```python
from build123d import *

# Parameters (mm, degrees)
BOSS_EXTRUDE1_DEPTH = 2


with BuildPart() as part:
    # Sketch1 → Boss-Extrude1 (new body)
    with BuildSketch(Plane(origin=(0, 0, 0), x_dir=(0, 0, -1), z_dir=(1, 0, 0))):
        with BuildLine():
            Line((-18, 0), (-15, 0))
            Line((-15, 0), (-15, 2))
            Line((-15, 2), (-5, 2))
            Line((-5, 2), (-5, 0))
            Line((-5, 0), (5, 0))
            Line((5, 0), (5, 2))
            Line((5, 2), (15, 2))
            Line((15, 2), (15, 0))
            Line((15, 0), (18, 0))
            Line((18, 0), (18, -2))
            Line((18, -2), (20, -2))
            Line((20, -2), (20, -12))
            Line((20, -12), (18, -12))
            Line((18, -12), (18, -15))
            ThreePointArc((18, -15), (0, -11.536096634), (-18, -15))
            Line((-18, -15), (-18, -12))
            Line((-18, -12), (-20, -12))
            Line((-20, -12), (-20, -2))
            Line((-20, -2), (-18, -2))
            Line((-18, -2), (-18, 0))
        make_face()
        with BuildLine():
            Line((-15, -12.339136563), (-15, -6))
            ThreePointArc((-15, -6), (-14.121320344, -3.878679656), (-12, -3))
            Line((-12, -3), (12, -3))
            ThreePointArc((12, -3), (14.121320344, -3.878679656), (15, -6))
            Line((15, -6), (15, -12.339136563))
            ThreePointArc((15, -12.339136563), (0, -10.036096634), (-15, -12.339136563))
        make_face(mode=Mode.SUBTRACT)
    extrude(amount=BOSS_EXTRUDE1_DEPTH)


solid = part.part
```
The listing builds one solid part. Answer for the finished solid, in the listing's coordinates (mm). A direction names the side the tool comes from. Give positions to 0.01 mm unless a question says otherwise; leave off trailing zeros. Order: outer loops, then holes, each group sorted by start corner. A loop starts at its lowest first (then second) coordinate and runs counter-clockwise, first axis right, second up. Notation, with made-up numbers: (78.25, -4.5) - (103.25, -4.5) arc R18 cw to (103.25, 2.5) - close; hole circle Ø8 at (-25.5, 67). An arc over 180 degrees is marked (long way). Use one line per item in the form item = value. Start each with the question number.
(1) The mould has two halves that part along Y. Classify faces 5 (the flat face through (1, -7, -20)), 6 (the flat face through (1, -9, -15)), 7 (the flat face through (1, -12, -19)), 8 (the flat face through (1, 2, -10)): released by +Y, released by -Y, zero draft, split by the parting line, or undercut.
(2) Consider line 1 (Z direction, x = 1.4, y = -7.25); line 2 (Z direction, x = 0.85, y = 0.5); line 3 (Y direction, x = 0.4, z = 18.5). Determine where each line is inside the solid, lowest interval first. Write a range as from..to.
(3) For faces 1 (the flat face through (1, -13, -18)), 2 (the flat face through (1, -1, -18)), 3 (the flat face through (1, 1, -5)), 4 (the cylindrical face through (0.99, -3.86, -14.1)), determine the directions among +Z, -Z, +X, -X, +Y, -Y from which every point of the face is accessible in a straight line to the end or side of a thin tool.
(4) A cutting plane is placed at A-A, the plane z = 0. Write down the section's boundary in (x, y), then the cut area to 3 significant figures.
(5) Flat-ended cylindrical pins translate along their axes: pin 1 Ø1 at (x, z) = (1, -0.5) entering from +Y; pin 2 Ø0.6 at (x, z) = (1, -19.5) entering from -Y; pin 3 Ø5 at (y, z) = (0.5, -15) entering from -X; pin 4 Ø0.6 at (x, y) = (1.5, 1.5) entering from -Z. Find the tip coordinate at first contact, or state that the pin passes through.
(6) A cutting plane is placed at B-B, the plane x = 1.1. Write down the section's boundary in (y, z).
(7) A cutting plane is placed at C-C, the plane y = -8.5. Write down the section's boundary in (x, z).
Ans:
q1.face_5 = zero draft
q1.face_6 = undercut
q1.face_7 = released by -Y
q1.face_8 = released by +Y
q2.line_1 = -20..-15, 15..20
q2.line_2 = -15..-5, 5..15
q2.line_3 = -12..-2
q3.face_1 = -Z, +X, -X, -Y
q3.face_2 = -Z, +X, -X, +Y
q3.face_3 = +X, -X, +Y
q3.face_4 = +X, -X
q4.outline = (0, -11.54) - (2, -11.54) - (2, -10.04) - (0, -10.04) - close; (0, -3) - (2, -3) - (2, 0) - (0, 0) - close
q4.area = 9.00 mm^2
q5.pin_1 = 0
q5.pin_2 = -12
q5.pin_3 = 0
q5.pin_4 = -15
q6.outline = (-15, -18) - (-12, -18) - (-12, -20) - (-2, -20) - (-2, -18) - (0, -18) - (0, -15) - (2, -15) - (2, -5) - (0, -5) - (0, 5) - (2, 5) - (2, 15) - (0, 15) - (0, 18) - (-2, 18) - (-2, 20) - (-12, 20) - (-12, 18) - (-15, 18) arc R48.5 cw to start; hole (-12.34, -15) - (-6, -15) arc R3 ccw to (-3, -12) - (-3, 12) arc R3 ccw to (-6, 15) - (-12.34, 15) arc R50 cw to start
q7.outline = (0, -20) - (2, -20) - (2, -15) - (0, -15) - close; (0, 15) - (2, 15) - (2, 20) - (0, 20) - close
